CAD build for the part. Positions are in the model's coordinates, mm. A direction names the side the tool comes from. Coordinates: 2 decimals unless noted, no trailing zeros. Loops run counter-clockwise (first coordinate to the right, second up) from the corner with the lowest first, then second, coordinate; pieces in that order, holes last.
1) Which spindle directions (+Z, -Z, +X, -X, +Y, -Y) get a long thin tool onto all of the face, cutting with end or side? Do faces 4 (the cylindrical face through (-1.115, -33.838, -1.216)), 5 (the flat face through (-3.045, 0.56, 1.726)), 6 (the cylindrical face through (-1.115, 33.838, -1.216)). Say none if no direction does.
2) Saw through at C-C, the plane x = 3. Write the cut outline in (y, z), and give its area (3 significant figures).
3) Saw through at A-A, the plane y = 35. Write the cut outline in (x, z).
4) Wall check: line 1 along X through (y, z) = (35.5, 0); line 2 along Z through (x, y) = (0, 31); line 3 along X through (y, z) = (25.5, -1.5). Give the ranges that are in metal, low to high.
5) Pin check, flat tips, straight feed: pin 1 Ø3 at (y, z) = (12.5, 0.5) entering from +X; pin 2 Ø2 at (x, z) = (0, 0) entering from +Y. Stop position of each tip, or through.
6) Saw through at B-B, the plane y = -11. Write the cut outline in (x, z), and give its area (3 significant figures).
7) Saw through at D-D, the plane z = 2.5. Write the cut outline in (x, y).
8) Two-plate mould, pull along Z, no slides. Class faces 1 (the flat face through (2, 40, 0)), 2 (the conical face through (0.1, -26.7, 0.3)), 3 (the flat face through (-3, 0.6, -1.8)): +Z half, -Z half, draft (parallel to the pull), parting line (faces both ways), or undercut.
```python
from build123d import *

# Parameters (mm, degrees)
SALIENTE_EXTRUIR1_DEPTH = 40


with BuildPart() as part:
    # Croquis1 → Saliente-Extruir1 (new, symmetric)
    with BuildSketch(Plane(origin=(0, 0, 0), x_dir=(1, 0, 0), z_dir=(0, 1, 0))):
        Polygon((-2.020725942, 3.5), (-4.041451884, 0), (-2.020725942, -3.5), (2.020725942, -3.5), (4.041451884, 0), (2.020725942, 3.5), align=None)
    extrude(amount=SALIENTE_EXTRUIR1_DEPTH, both=True)

    # Croquis4 → Taladro roscado M41 (revolve, cut)
    with BuildSketch(Plane(origin=(0, 40, 0), x_dir=(0, 0, 1), z_dir=(1, 0, 0))):
        Polygon((0, 0), (0, 13.491420021), (1.65, 12.5), (1.65, 0), align=None)
    taladro_roscado_m41 = revolve(axis=Axis((0, 46.35, 0), (0, -1, 0)), mode=Mode.SUBTRACT)

    # Simetría1: Taladro roscado M41 across plane
    add(taladro_roscado_m41.mirror(Plane.ZX), mode=Mode.SUBTRACT)


solid = part.part
```
Data:
1. face 4: -Y
1. face 5: +Z, -X, +Y, -Y
1. face 6: +Y
2. outline: (-40, -1.8) - (40, -1.8) - (40, 1.8) - (-40, 1.8) - close
2. area: 289 mm2
3. outline: (-4.04, 0) - (-2.02, -3.5) - (2.02, -3.5) - (4.04, 0) - (2.02, 3.5) - (-2.02, 3.5) - close; hole circle Ø3.3 at (0, 0)
4. line 1: x = -4.04 to -1.65, 1.65 to 4.04
4. line 2: z = -3.5 to -1.65, 1.65 to 3.5
4. line 3: x = -3.18 to 3.18
5. pin 1: stops at x = 4.04
5. pin 2: stops at y = 27.11
6. outline: (-4.04, 0) - (-2.02, -3.5) - (2.02, -3.5) - (4.04, 0) - (2.02, 3.5) - (-2.02, 3.5) - close
6. area: 42.4 mm2
7. outline: (-2.6, -40) - (2.6, -40) - (2.6, 40) - (-2.6, 40) - close
8. face 1: draft
8. face 2: undercut
8. face 3: -Z half
